The model under review builds one solid part; all positions refer to its coordinate system, in mm. Face numbers are marked on the shaded views. A direction names the side the tool comes from. Round coordinates to 2 decimals unless told otherwise and drop trailing zeros. Order: outer loops, then holes, each group sorted by start corner. A loop starts at its lowest first (then second) coordinate and runs counter-clockwise, first axis right, second up.
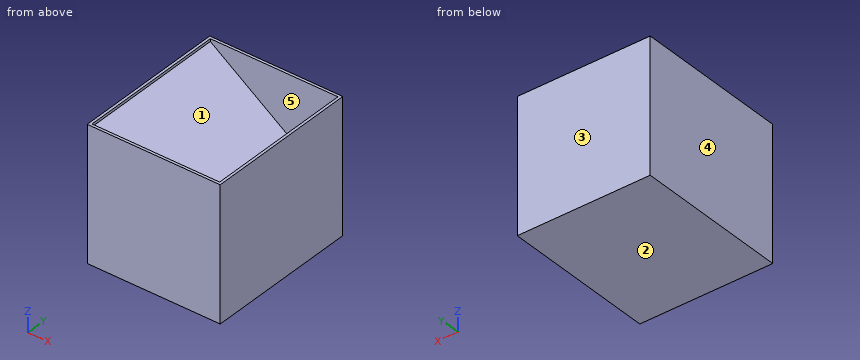
```python
from build123d import *

# Parameters (mm, degrees)
SKETCH_W     = 250
SKETCH_H     = 290
PAD_DEPTH    = 250
SKETCH002_W  = 240
SKETCH002_H  = 280
POCKET_DEPTH = 240
PAD001_DEPTH = 290


with BuildPart() as part:
    # Sketch → Pad (new body)
    with BuildSketch(Plane.XY):
        Rectangle(SKETCH_W, SKETCH_H)
    extrude(amount=PAD_DEPTH)

    # Sketch002 (on Face6 of Pad) → Pocket (cut)
    with BuildSketch(Plane.XY.offset(250)):
        Rectangle(SKETCH002_W, SKETCH002_H)
    extrude(amount=-POCKET_DEPTH, mode=Mode.SUBTRACT)

    # Sketch003 (on Face1 of Pocket) → Pad001 (join)
    with BuildSketch(Plane.XZ.offset(145)):
        Polygon((-120, 245), (-120, 5), (120, 5), (120, 72.606014), align=None)
    extrude(amount=-PAD001_DEPTH)


solid = part.part
```
(1) For the marked faces 1 and 2, list the 3-axis set-ups (+Z, -Z, +X, -X, +Y, -Y) from which the entire face can be reached by the end or side of a thin tool; tool diameter is ignored.
Data:
face 1: +Z
face 2: -Z, +X, -X, +Y, -Y
(2) Consider section D-D (z = 98). Write out the cut boundary in (x, y), and give its area (3 significant figures).
Data:
outline: (-125, -145) - (125, -145) - (125, 145) - (-125, 145) - close; hole (84.65, -140) - (120, -140) - (120, 140) - (84.65, 140) - close
area: 62,600 mm2
(3) Consider section C-C (z = 191). Write out the cut boundary in (x, y), and give its area (3 significant figures).
Data:
outline: (-125, -145) - (125, -145) - (125, 145) - (-125, 145) - close; hole (-44.82, -140) - (120, -140) - (120, 140) - (-44.82, 140) - close
area: 26,300 mm2
(4) Consider section B-B (x = -48.5). Write out the cut boundary in (y, z).
Data:
outline: (-145, 0) - (145, 0) - (145, 250) - (140, 250) - (140, 193.64) - (-140, 193.64) - (-140, 250) - (-145, 250) - close
(5) Insertion check: pin 1 (6 mm diameter, centred on x = -84.5, y = 6, fed in from +Z) (3 decimals); pin 2 (6 mm diameter, centred on x = -2, y = 75, fed in from +Z); pin 3 (5 mm diameter, centred on x = 50.5, y = 104.5, fed in from +Z). Each pin has a flat end and moves straight along its axis. Give the tip position at first contact, or say it passes through.
Data:
pin 1: stops at z = 221.655
pin 2: stops at z = 162.39
pin 3: stops at z = 124.32
(6) Draft analysis for pull direction Y (two halves, no side actions). For the marked faces 3, 4 and 5, state which applies: pulls with the +Y half, pulls with the -Y half, needs draft (parallel to the pull), parting line crosses it, or undercut.
Data:
face 3: pulls with the +Y half
face 4: needs draft
face 5: undercut
(7) Consider section A-A (y = 14.5). Write out the cut boundary in (x, z).
Data:
outline: (-125, 0) - (125, 0) - (125, 250) - (120, 250) - (120, 72.61) - (-120, 245) - (-120, 250) - (-125, 250) - close
(8) To check wall thickness, follow probe 1 along Y at (x, z) = (69, 131.5); probe 2 along X at (y, z) = (50.5, 150); probe 3 along X at (y, z) = (1.5, 97). State the ranges of each line that lie inside material, in increasing order.
Data:
probe 1: y = -145 to -140, 140 to 145
probe 2: x = -125 to 12.26, 120 to 125
probe 3: x = -125 to 86.04, 120 to 125
